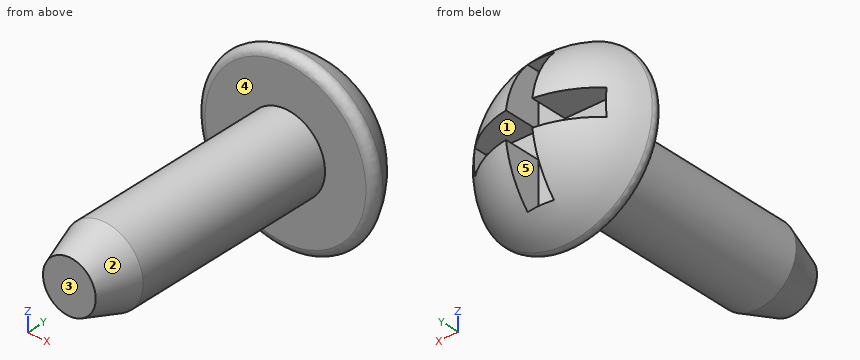
from build123d import *

# Parameters (mm, degrees)
FILLET1_R          = 0.3
CUT_EXTRUDE1_START = 1
CUT_EXTRUDE1_DEPTH = 10.616564891


with BuildPart() as part:
    # Sketch1 → Revolve1 (revolve)
    with BuildSketch(Plane.XY, mode=Mode.PRIVATE) as revolve1_sk:
        with BuildLine():
            Line((-1.5, 0), (-1.5, -8))
            Line((-1.5, -8), (-1, -9.5))
            Line((-1, -9.5), (0, -9.5))
            Line((0, -9.5), (0, 2.5))
            ThreePointArc((0, 2.5), (-2.150581317, 1.810813843), (-3.5, 0))
            Line((-3.5, 0), (-1.5, 0))
        make_face()
    revolve(revolve1_sk.sketch.rotate(Axis((0, -2.514017632, 0), (0, -1, 0)), 270), axis=Axis((0, -2.514017632, 0), (0, -1, 0)))

    # Fillet1
    fillet1_edges = [part.edges().sort_by_distance(p)[0] for p in [
        (0, 0, -3.5),
    ]]
    fillet(fillet1_edges, radius=FILLET1_R)

    # Sketch2 → Cut-Extrude1 (cut, through all)
    with BuildSketch(Plane(origin=(0, 0, 0), x_dir=(1, 0, 0), z_dir=(0, 1, 0)).offset(CUT_EXTRUDE1_START)):
        Polygon((0.5, 0.5), (2.5, 0.5), (2.5, -0.5), (0.5, -0.5), (0.5, -2.5), (-0.5, -2.5), (-0.5, -0.5), (-2.5, -0.5), (-2.5, 0.5), (-0.5, 0.5), (-0.5, 2.5), (0.5, 2.5), align=None)
    extrude(amount=CUT_EXTRUDE1_DEPTH, mode=Mode.SUBTRACT)


solid = part.part
Work out the finished part from the listing and answer in its coordinate system (mm). Face numbers are marked on the shaded views. A direction names the side the tool comes from. Coordinates: 2 decimals unless noted, no trailing zeros. Write each loop counter-clockwise with the first axis right and the second up, starting at its lowest first coordinate (ties: lowest second). Pieces come first, ordered by that corner, then holes. Notation, with made-up numbers: M 7,85 L 29,85 A17 ccw 29,111 Z; hole C -9,-28.5 d9. An arc over 180 degrees is marked long. Write item = value, one per line.
1. Flat-ended cylindrical pins translate along their axes: pin 1 (4 mm diameter, centred on x = 2.5, z = -1.5, fed in from +Y); pin 2 (2 mm diameter, centred on y = -3.5, z = -0.5, fed in from +X); pin 3 (0.6 mm diameter, centred on x = 0, y = 1.5, fed in from +Z). Find the tip coordinate at first contact, or state that the pin passes through.
Solution:
pin_1 = 2.38
pin_2 = 1.5
pin_3 = 2.82
2. The part is cut by section A-A (y = -2). Determine the outline of the cut face in (x, z), then the cut area to 3 significant figures.
Solution:
outline = C 0,0 d3
area = 7.07 mm2
3. Straight lines are drawn through the part: line 1 (Y direction, x = 1.75, z = -0.25); line 2 (Z direction, x = -2, y = 1.25); line 3 (Y direction, x = -0.25, z = 0). For each, find the intervals that lie inside material, in ascending order. Write a range as from..to.
Solution:
line_1 = 0..1
line_2 = -1.92..-0.5, 0.5..1.92
line_3 = -9.5..1
4. For the marked faces 4 and 5, determine the directions among +Z, -Z, +X, -X, +Y, -Y from which every point of the face is accessible in a straight line to the end or side of a thin tool.
Solution:
face_4 = -Y
face_5 = +Y
5. Determine the mould class of the marked faces 1, 2 and 3 for opening direction Z: released by +Z, released by -Z, zero draft, split by the parting line, or undercut.
Solution:
face_1 = undercut
face_2 = split by the parting line
face_3 = zero draft
